Check sheet for the modelled part. Datum: model origin and axes. Units: mm. Face numbers are marked on the shaded views. A direction names the side the tool comes from. Round coordinates to 2 decimals unless told otherwise and drop trailing zeros. Write each loop counter-clockwise with the first axis right and the second up, starting at its lowest first coordinate (ties: lowest second). Pieces come first, ordered by that corner, then holes. Notation, with made-up numbers: (-12.75, -38) - (7.25, -38) arc R11 ccw to (7.25, -31) - close; hole circle Ø2 at (53, -19). An arc over 180 degrees is marked (long way). Answer as a JSON object with one key per item and string values. Group by question number.
Item 1: Sectioned sample at C-C on y = 1.2. Record the boundary of the cut face in (x, z), plus the area to 4 significant figures.
Item 2: Sectioned sample at A-A on z = 0.5. Record the boundary of the cut face in (x, y), plus the area to 3 significant figures.
Item 3: Sectioned sample at D-D on x = 1.5. Record the boundary of the cut face in (y, z).
Item 4: Thickness scan on line 1 (X direction, y = 0.45, z = -9.5); line 2 (Z direction, x = -2, y = -2.8); line 3 (Y direction, x = 2, z = -4.5). Record the ranges inside material, lowest first.
Item 5: Set-up check for the marked faces 1, 2 and 3: record each of +Z, -Z, +X, -X, +Y, -Y from which the full face is reachable in a straight line by a thin tool's end or side.
Item 6: Gauge pin test, flat ends, axial feed: P1, Ø1.4, axis at y = 0, z = -3.5, coming from the +X side; P2, Ø1.2, axis at y = 1, z = 4.5, coming from the -X side; P3, Ø0.9, axis at x = 1, y = -3.5, coming from the +Z side. Record the tip position at first contact, or that the pin passes through.
Item 7: Sectioned sample at B-B on x = -4.5. Record the boundary of the cut face in (y, z), plus the area to 3 significant figures.
Autodesk Inventor part; units mm, degrees
ref_plane "YZ Plane" through (0, 0, 0) normal (1, 0, 0) x (0, 1, 0)
ref_plane "XZ Plane" through (0, 0, 0) normal (0, 1, 0) x (-1, 0, 0)
ref_plane "XY Plane" through (0, 0, 0) normal (0, 0, 1) x (1, 0, 0)
sketch "Sketch1" plane through (0, 0, 0) normal (0, 1, 0) x (-1, 0, 0)
  line L0 (0.85, 10.55) -> (-0.85, 10.55)
  line L1 (-0.85, 10.55) -> (-0.85, -10.55)
  line L2 (-0.85, -10.55) -> (0.85, -10.55)
  line L3 (0.85, -10.55) -> (0.85, 10.55)
  line L4 (0.85, 10.55) -> (-0.85, -10.55) construction
  line L5 (-0.85, 10.55) -> (0.85, -10.55) construction
  line L6 (2.35, 12.05) -> (-2.35, 12.05)
  line L7 (-2.35, 12.05) -> (-2.35, -12.05)
  line L8 (-2.35, -12.05) -> (2.35, -12.05)
  line L9 (2.35, -12.05) -> (2.35, 12.05)
  point P0 (0, 0)
  dimension "d0" = 1.7
  dimension "d1" = 21.1
  dimension "d2" = 1.5
extrude "Extrusion1" add sketch "Sketch1" along normal blind 1.5
sketch "Sketch2" plane through (0, 0, 0) normal (0, -1, 0) x (1, 0, 0)
  line L0 (4.95, 12.05) -> (-6.05, 12.05)
  line L1 (-6.05, 12.05) -> (-6.05, -12.05)
  line L2 (-6.05, -12.05) -> (4.95, -12.05)
  line L3 (4.95, -12.05) -> (4.95, 12.05)
  line L4 (-2.35, 12.05) -> (2.35, 12.05)
  line L5 (-2.35, -12.05) -> (-2.35, 12.05)
  dimension "d5" = 11
  dimension "d6" = 3.7
extrude "Extrusion2" add sketch "Sketch2" along normal blind 2.4
sketch "Sketch3" plane through (0, 0, 0) normal (0, 1, 0) x (1, 0, 0)
  line L0 (-2.35, 12.05) -> (-2.35, -12.05)
  line L1 (-6.05, 12.05) -> (-2.35, 12.05)
  line L2 (-6.05, -12.05) -> (-6.05, 12.05)
  line L3 (-2.35, -12.05) -> (-6.05, -12.05)
  line L4 (2.35, -12.05) -> (2.35, 12.05)
  line L5 (4.95, -12.05) -> (2.35, -12.05)
  line L6 (4.95, 12.05) -> (4.95, -12.05)
  line L7 (2.35, 12.05) -> (4.95, 12.05)
  point P0 (0, 0)
extrude "Extrusion3" cut sketch "Sketch3" against normal blind 1.4
move faces "Move1" translate (0, 0, -1.5) faces at (0.7833, 0.5333, 12.05)
sketch "Sketch4" plane through (0, -2.4, 0) normal (0, -1, 0) x (1, 0, 0)
  line L0 (-0.85, -10.55) -> (0.85, -10.55)
  line L1 (-6.05, 10.55) -> (-6.05, -12.05)
  line L2 (2.35, -12.05) -> (4.95, -12.05)
  line L3 (-6.05, -10.55) -> (4.95, -10.55)
  line L4 (4.95, -10.55) -> (4.95, -12.05)
  line L5 (4.95, -12.05) -> (-6.05, -12.05)
  line L6 (-6.05, -12.05) -> (-6.05, -10.55)
  point P0 (0, 0)
extrude "Extrusion4" add sketch "Sketch4" along normal blind 1.8
properties part number "gyro_holder"
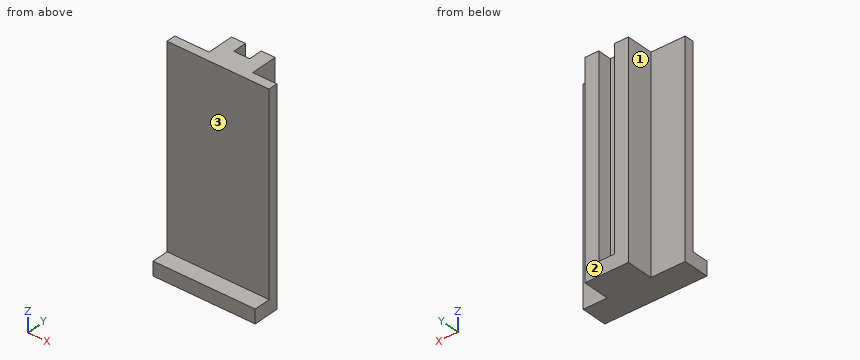
Completed:
{
 "1": {"outline": "(-2.35, -12.05) - (2.35, -12.05) - (2.35, 10.55) - (0.85, 10.55) - (0.85, -10.55) - (-0.85, -10.55) - (-0.85, 10.55) - (-2.35, 10.55) - close", "area": "70.35 mm²"},
 "2": {"outline": "(-6.05, -2.4) - (4.95, -2.4) - (4.95, -1.4) - (2.35, -1.4) - (2.35, 1.5) - (0.85, 1.5) - (0.85, 0) - (-0.85, 0) - (-0.85, 1.5) - (-2.35, 1.5) - (-2.35, -1.4) - (-6.05, -1.4) - close", "area": "22.1 mm²"},
 "3": {"outline": "(-4.2, -12.05) - (1.5, -12.05) - (1.5, 10.55) - (-2.4, 10.55) - (-2.4, -10.55) - (-4.2, -10.55) - close"},
 "4": {"line 1": "-2.35 to -0.85, 0.85 to 2.35", "line 2": "-12.05 to -10.55", "line 3": "-2.4 to 1.5"},
 "5": {"face 1": "+Z, -Z, -X, +Y", "face 2": "+Z, -Z, +X, -X, +Y", "face 3": "+Z, +X, -X, -Y"},
 "6": {"P1": "x = 2.35", "P2": "x = -2.35", "P3": "z = -10.55"},
 "7": {"outline": "(-4.2, -12.05) - (-1.4, -12.05) - (-1.4, 10.55) - (-2.4, 10.55) - (-2.4, -10.55) - (-4.2, -10.55) - close", "area": "25.3 mm²"}
}
